Build history of the part. All positions in model axes, mm. Round coordinates to 2 decimals unless told otherwise and drop trailing zeros. Loops run counter-clockwise (first coordinate to the right, second up) from the corner with the lowest first, then second, coordinate; pieces in that order, holes last. Notation, with made-up numbers: (22, 69.25) - (47, 69.25) arc R3 ccw to (47, 74.25) - close; hole circle Ø7 at (-21, 16). An arc over 180 degrees is marked (long way). Use a Markdown table: item, result.
Autodesk Inventor part; units mm, degrees
ref_plane "Work Plane1" through (187.0611, 458.9587, 0) normal (0, 0, 1) x (0.1591916, 0.9872477, 0)
ref_plane "YZ Plane" through (0, 0, 0) normal (1, 0, 0) x (0, 1, 0)
ref_plane "XZ Plane" through (0, 0, 0) normal (0, 1, 0) x (-1, 0, 0)
ref_plane "Work Plane1" through (187.0611, 458.9587, 0) normal (0, 0, 1) x (0.1591916, 0.9872477, 0)
sketch "Sketch1" plane through (187.0611, 458.9587, 0) normal (0, 0, 1) x (0.1591916, 0.9872477, 0)
  line L0 (5.0953, 0.0423) -> (5.0108, 609.6423)
  line L1 (-36.1797, 0.0366) -> (-36.2642, 609.6366)
  line L2 (-87.0268, 299.6189) -> (-40.0368, 299.6189)
  line L3 (5.0667, 206.0736) -> (-239.4228, 300.8893)
  line L4 (-87.0268, 401.2189) -> (-239.4268, 401.2189)
  line L5 (5.0265, 496.0682) -> (-239.4268, 401.2189)
  circle A0 centre (-207.6768, 350.4189) radius 15.4305 construction
  circle A1 centre (-207.6768, 350.4189) radius 13.0556 construction
  circle A2 centre (-207.6767, 351.037) radius 12.7
  line L6 (5.0466, 351.0648) -> (-194.9767, 351.037)
  line L7 (-220.3767, 351.037) -> (-239.4267, 351.037)
  line L8 (-239.4267, 351.037) -> (-239.4267, 325.637)
  line L9 (-239.4267, 351.037) -> (-239.4267, 376.437)
  line L10 (-239.4267, 325.637) -> (5.0537, 300.2648)
  line L11 (-239.4267, 376.437) -> (5.0396, 401.8648)
  point P0 (-482.8845, 111.6133)
  point P1 (5.0526, 307.6736)
  point P2 (5.0406, 394.4682)
  point P3 (5.0304, 467.7016)
  point P4 (5.0628, 234.4154)
  point P5 (-239.4268, 372.8507)
  dimension "d0" = 101.6
  dimension "d1" = 101.6
  dimension "d2" = 233.2861
  dimension "d30" = 244.4764
  dimension "d35" = 25.4
  dimension "d38" = 25.4
  dimension "d39" = 25.4
  dimension "d40" = 200.0234
  dimension "d41" = 50.8
  dimension "d42" = 50.8
  dimension "d43" = 19.05
  dimension "d44" = 25.4277
  dimension "d45" = 25.3723
extrude "Plate1" add sketch "Sketch1" along normal blind 3.048 contours L10 L1 L6 L0 | L6 L1 L11 L0 | L10 L8 L7 A2 L6 L1 | L6 A2 L7 L9 L11 L1
sketch "Sketch2" plane through (187.0611, 458.9587, 3.048) normal (0, 0, 1) x (0.1591916, 0.9872477, 0)
  circle A0 centre (-195.4493, 362.9394) radius 2.1463
  circle A1 centre (-220.1972, 362.6464) radius 2.1463
  circle A2 centre (-219.9042, 337.8985) radius 2.1463
  circle A3 centre (-195.1563, 338.1915) radius 2.1463
  point P0 (-482.8845, 111.6133)
extrude "Extrusion1" cut sketch "Sketch2" against normal up to surface (3.048 mm away)
sketch "Sketch3" plane through (187.0611, 458.9587, 3.048) normal (0, 0, 1) x (0.1591916, 0.9872477, 0)
  circle A0 centre (-207.6767, 351.037) radius 12.7
  circle A1 centre (-207.6767, 351.037) radius 13.4937
  point P0 (-482.8845, 111.6133)
  point P1 (-207.6768, 350.4189)
  dimension "d36" = 0.7937
extrude "Extrusion2" cut sketch "Sketch3" against normal up to surface (3.048 mm away)
sketch "Sketch5" plane through (187.0611, 458.9587, 3.048) normal (0, 0, 1) x (0.9872477, -0.1591916, 0)
  line L0 (-401.8648, 5.0396) -> (-300.2648, 5.0537)
  line L1 (-300.2648, 5.0537) -> (-401.8648, 5.0396) construction
  line L2 (-319.3169, 5.051) -> (-319.3151, -7.649) construction
  line L3 (-401.8648, 5.0396) -> (-376.437, -239.4267)
  line L4 (-319.3151, -7.649) -> (-301.583, -7.649)
  line L5 (-300.2648, 5.0537) -> (-325.637, -239.4267)
  circle A0 centre (-376.4648, -7.649) radius 3.175
  circle A1 centre (-325.6648, -7.649) radius 3.175
  line L6 (-319.3151, -7.649) -> (-322.4898, -7.649)
  line L7 (-328.8398, -7.649) -> (-373.2898, -7.649)
  line L8 (-379.6398, -7.649) -> (-400.545, -7.649)
  point P0 (-111.6133, -482.8845)
  point P1 (-351.0648, 5.0466)
  dimension "d47" = 12.7
  dimension "d48" = 12.7025
  dimension "d49" = 6.35
  dimension "d50" = 6.35
  dimension "d51" = 50.8
  dimension "d52" = 50.8
  dimension "d53" = 25.4
sketch "Sketch6" plane through (187.0611, 458.9587, 0) normal (0, 0, -1) x (-0.9872477, 0.1591916, 0)
  circle A0 centre (337.8985, -219.9042) radius 2.1463
  circle A1 centre (338.1915, -195.1563) radius 2.1463
  circle A2 centre (362.6464, -220.1972) radius 2.1463
  circle A3 centre (362.9394, -195.4493) radius 2.1463
  line L0 (325.637, -239.4267) -> (376.437, -239.4267)
  line L1 (300.2648, 5.0537) -> (325.637, -239.4267)
  line L2 (376.437, -239.4267) -> (401.8648, 5.0396)
  line L3 (401.8648, 5.0396) -> (300.2648, 5.0537)
  circle A4 centre (338.337, -172.7517) radius 2.9337
  circle A5 centre (338.337, -141.0017) radius 2.9337
  circle A6 centre (363.737, -141.0017) radius 2.9337
  circle A7 centre (363.737, -172.7517) radius 2.9337
  circle A8 centre (338.337, -109.2517) radius 2.9337
  circle A9 centre (363.737, -109.2517) radius 2.9337
  point P0 (111.6133, -482.8845)
extrude "Extrusion5" cut sketch "Sketch6" against normal up to next contours A4 | A5 | A6 | A7 | A8 | A9
sketch "Sketch7" plane through (187.0611, 458.9587, 0) normal (0, 0, -1) x (-0.9872477, 0.1591916, 0)
  circle A0 centre (367.9532, -233.0767) radius 2.54
  circle A1 centre (349.8669, -233.0767) radius 2.54
  point P0 (111.6133, -482.8845)
extrude "Extrusion6" cut sketch "Sketch7" against normal up to next
extrude "Extrusion7" cut sketch "Sketch5" against normal up to next contours A0 | A1
fillet "Fillet1" radius 12.7 2 edges at (-108.57, 511.7476, 1.524) (-208.8766, 527.9075, 1.524)
fillet "Fillet2" radius 6.35 2 edges at (-222.6902, 282.5108, 1.524) (-172.538, 274.4239, 1.524)
equation "\"BendRadius\" = Thickness"
equation "\"BendReliefWidth\" = Thickness"
equation "\"BendReliefDepth\" = 0.5 * Thickness"
equation "\"CornerReliefSize\" = 4 * Thickness"
equation "\"MinimumRemnant\" = 2 * Thickness"
equation "\"TransitionRadius\" = BendRadius"
equation "\"JacobiRadiusSize\" = BendRadius"
equation "\"GapSize\" = Thickness"
equation "\"d4\" = BendRadius"
properties part number "lifterMountMetal"
Q1. Cut at D-D, the plane y = 485. List the corners of the cut face in (x, z).
Results found:
| item | result |
|---|---|
| outline | (-211.29, 0) - (-115.78, 0) - (-115.78, 3.05) - (-211.29, 3.05) - close |
Q2. Cut at C-C, the plane x = -156. List the corners of the cut face in (y, z), plus the area to 3 significant figures.
Results found:
| item | result |
|---|---|
| outline | (335.78, 0) - (519.39, 0) - (519.39, 3.05) - (335.78, 3.05) - close |
| area | 560 mm2 |
Q3. Probe line 1 (Y direction, x = -195.5, z = 0.3); line 2 (Y direction, x = -181, z = 1.25); line 3 (X direction, y = 298.5, z = 2.15). List the from-to ranges inside material, lowest first.
Results found:
| item | result |
|---|---|
| line 1 | y = 278.13 to 282.01, 287.09 to 296.64, 322.98 to 374.91, 380.41 to 525.74 |
| line 2 | y = 275.79 to 293.57, 297.73 to 302.85, 316.77 to 523.42 |
| line 3 | x = -221.79 to -208.01, -204.02 to -199.92, -185.2 to -166.05 |
Q4. Pull direction X, two halves, no side cores. Call faces 1 (the face through (-211.56, 285.58, 1.5)), 2 (the face through (-197.89, 278.51, 1.5)), 3 (the face through (-178.2, 322.25, 1.55)), 4 (the face through (-142.054, 387.521, 1.503)): pulls with the +X half, pulls with the -X half, needs draft (parallel to the pull), parting line crosses it, or undercut.
Results found:
| item | result |
|---|---|
| face 1 | undercut |
| face 2 | pulls with the -X half |
| face 3 | undercut |
| face 4 | pulls with the +X half |
Q5. Drop flat-ended pins along their axis: pin 1 (21.5 mm diameter, centred on x = -192.56, y = 309.81, fed in from +Z); pin 2 (1.5 mm diameter, centred on x = -202, z = 0.5, fed in from +Y). Give the stop position or say it passes through.
Results found:
| item | result |
|---|---|
| pin 1 | passes through |
| pin 2 | stops at y = 525.09 |
Q6. Cut at B-B, the plane y = 310. List the corners of the cut face in (x, z), plus the area to 3 significant figures.
Results found:
| item | result |
|---|---|
| outline | (-221.14, 0) - (-206.05, 0) - (-206.05, 3.05) - (-221.14, 3.05) - close; (-179.07, 0) - (-162.95, 0) - (-162.95, 3.05) - (-179.07, 3.05) - close |
| area | 95.1 mm2 |
